Answer from the drawing. Dimensions are ordinates in mm from the lowest x, y and z of the part. Round coordinates to 2 decimals unless told otherwise and drop trailing zeros. Loops run counter-clockwise (first coordinate to the right, second up) from the corner with the lowest first, then second, coordinate; pieces in that order, holes last. Notation, with made-up numbers: M -16.5,59 L -11.5,59 A22 cw -11.5,97 Z; hole C -22.75,11.25 d10. An arc over 180 degrees is marked long. One line per item, written item: value.
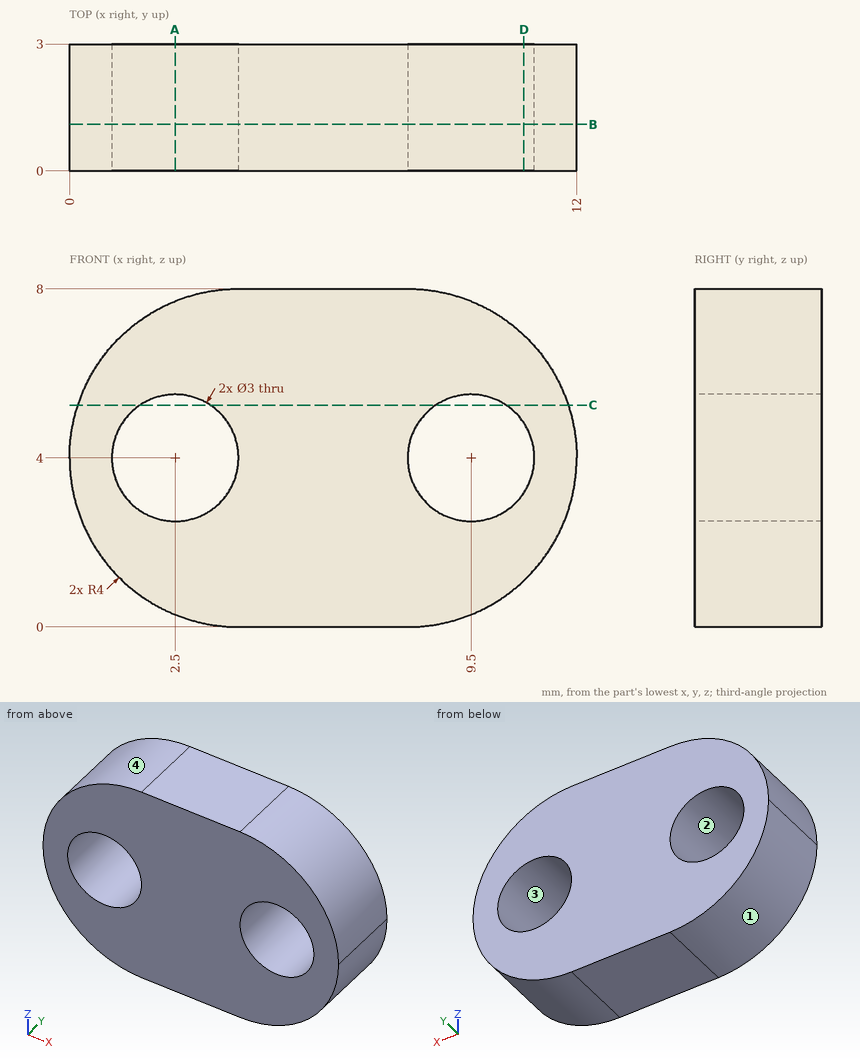
1) Find the intervals of material crossed by probe 1 along X at (y, z) = (0.85, 4.5); probe 2 along X at (y, z) = (0.9, 3.25); probe 3 along Z at (x, y) = (9.75, 1.05), in increasing order. Write a range as from..to.
Check values:
probe 1: 0.03..1.09, 3.91..8.09, 10.91..11.97
probe 2: 0.07..1.2, 3.8..8.2, 10.8..11.93
probe 3: 0.4..2.52, 5.48..7.6
2) Find section D-D (x = 10.75). Give the vertices of the cut face in (y, z), then the cut area to 3 significant figures.
Check values:
outline: M 0,1.1 L 3,1.1 L 3,3.17 L 0,3.17 Z; M 0,4.83 L 3,4.83 L 3,6.9 L 0,6.9 Z
area: 12.5 mm2
3) Find section B-B (y = 1.1). Give the number of separate pieces and of enclosed holes in the cut face, then the cut area to 3 significant figures.
Check values:
separate pieces: 1
enclosed holes: 2
area: 68.1 mm2
4) The mould has two halves that part along Z. Classify the marked faces 1, 2, 3 and 4: +Z half, -Z half, draft (parallel to the pull), parting line (faces both ways), or undercut.
Check values:
face 1: -Z half
face 2: undercut
face 3: undercut
face 4: +Z half
5) Find section A-A (x = 2.5). Give the vertices of the cut face in (y, z), then the cut area to 3 significant figures.
Check values:
outline: M 0,0.29 L 3,0.29 L 3,2.5 L 0,2.5 Z; M 0,5.5 L 3,5.5 L 3,7.71 L 0,7.71 Z
area: 13.2 mm2
6) Find section C-C (z = 5.25). Give the vertices of the cut face in (x, y).
Check values:
outline: M 0.2,0 L 1.67,0 L 1.67,3 L 0.2,3 Z; M 3.33,0 L 8.67,0 L 8.67,3 L 3.33,3 Z; M 10.33,0 L 11.8,0 L 11.8,3 L 10.33,3 Z
